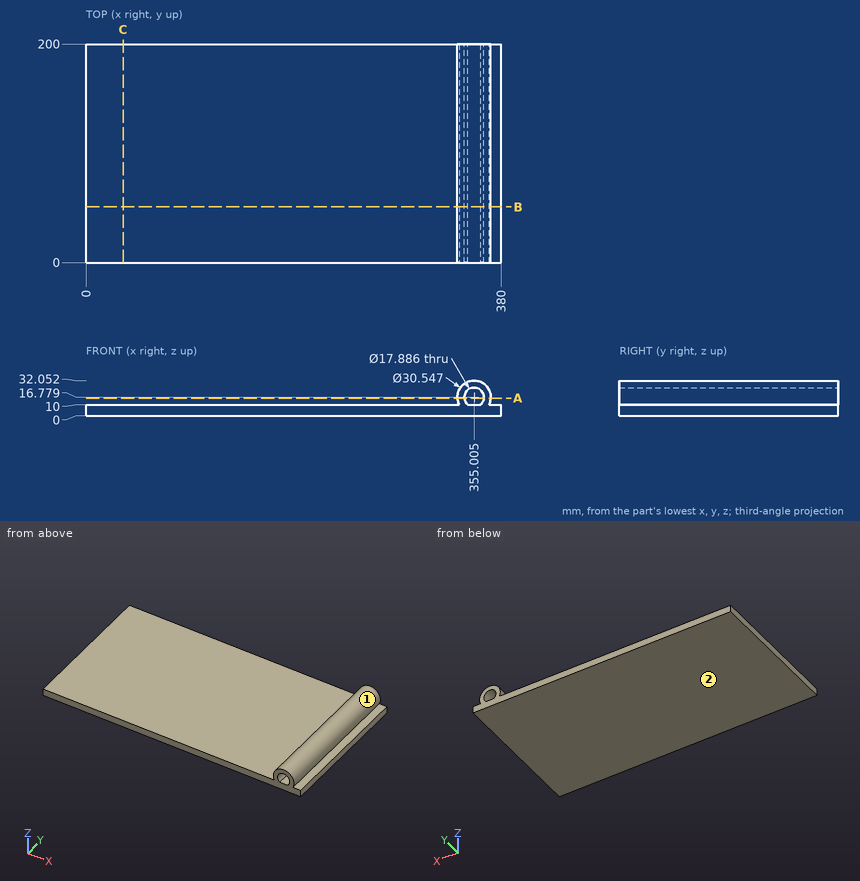
Could you check a few things on this drawing? It's one solid part, dimensions in mm from its lowest x, y, z. Round coordinates to 2 decimals unless told otherwise and drop trailing zeros. Order: outer loops, then holes, each group sorted by start corner. A loop starts at its lowest first (then second) coordinate and runs counter-clockwise, first axis right, second up. Notation, with made-up numbers: M 39.25,-36 L 79.25,-36 A6 ccw 79.25,-30 Z; hole C 18,81 d2. An arc over 180 degrees is marked long. Return JSON: item names as keys, results as strings. Group by question number.
1. If we mould it in two halves opening along Z, with no side actions, what happens to the marked faces 1 and 2? For each: pulls with the +Z half, pulls with the -Z half, needs draft (parallel to the pull), parting line crosses it, or undercut.
2. I'm going to push flat-ended pins straight in: pin 1 Ø3.5 at (x, y) = (373.5, 132) entering from +Z; pin 2 Ø3 at (y, z) = (35.5, 12) entering from -X; pin 3 Ø6 at (y, z) = (70, 18) entering from -X. Where does each tip first touch, or does it pass through?
3. If we section it at A-A on z = 16: List the corners of the cut face in (x, y) for me (1 decimal), then the cut area to 3 significant figures.
4. If we section it at C-C on x = 34: List the corners of the cut face in (y, z) for me.
5. Please list where these lines run through material, in increasing order: probe 1 along Z at (x, y) = (194, 104.5); probe 2 along X at (y, z) = (169, 24.5) (1 decimal); probe 3 along X at (y, z) = (50.5, 21) (1 decimal).
6. If we section it at B-B on y = 51: List the corners of the cut face in (x, z) for me (1 decimal).
Reply:
{
 "1": {"face 1": "undercut", "face 2": "pulls with the -Z half"},
 "2": {"pin 1": "z = 10", "pin 2": "x = 340.09", "pin 3": "x = 339.73"},
 "3": {"outline": "M 339.8,0 L 346.1,0 L 346.1,200 L 339.8,200 Z; M 363.9,0 L 370.3,0 L 370.3,200 L 363.9,200 Z", "area": "2,540 mm^2"},
 "4": {"outline": "M 0,0 L 200,0 L 200,10 L 0,10 Z"},
 "5": {"probe 1": "0 to 10", "probe 2": "341.8 to 350.5, 359.5 to 368.2", "probe 3": "340.3 to 347.1, 362.9 to 369.7"},
 "6": {"outline": "M 0,0 L 380,0 L 380,10 L 368.7,10 A15.3 ccw long 341.3,10 L 0,10 Z; hole M 349.2,10 L 360.8,10 A8.9 ccw long Z"}
}
